Could you check a few things on this model? Use its own coordinates, in mm. Round coordinates to 2 decimals unless told otherwise and drop trailing zeros. Write each loop counter-clockwise with the first axis right and the second up, starting at its lowest first coordinate (ties: lowest second). Pieces come first, ordered by that corner, then holes. Notation, with made-up numbers: M 34,43 L 84,43 A8 cw 84,52 Z; hole C -29,-29.75 d5. An arc over 180 degrees is marked long. One line per item, written item: value. Start each with the question number.
(1) I want a section at B-B on y = 459. Please give me the cut outline in (x, z).
(2) I'm going to push flat-ended pins straight in: pin 1 Ø8 at (x, y) = (88.9, 12.7) entering from -Z; pin 2 Ø3 at (y, z) = (639, 2) entering from +X. Where does each tip first touch, or does it pass through?
(3) If I drill on L1, parallel to X at y = 1714.5, z = 3.5; L2, parallel to Y at x = 571.5, z = 5; L3, parallel to Y at x = 304.8, z = 4.25, over which ranges is the centre line in solid material (lowest first)?
(4) I want a section at A-A on z = 4.25. Count the separate pieces of the cut face and the enclosed holes in it, and give its area (3 significant figures).
```python
from build123d import *

# Parameters (mm, degrees)
SKETCH2_W                                       = 584.2
SKETCH2_H                                       = 1727.2
BOSS_EXTRUDE1_DEPTH                             = 6.35
CUT_EXTRUDE1_DEPTH                              = 1824.334802635
H_0_266_DIAMETER_HOLE1_D                        = 6.7564
FILLET1_R                                       = 6.35
SKETCH7_R                                       = 3.3782
CUT_EXTRUDE2_DEPTH                              = 12.7
CSK_FOR_10_FLAT_HEAD_MACHINE_SCREW1_D           = 5.6134
CSK_FOR_10_FLAT_HEAD_MACHINE_SCREW1_CSINK_D     = 9.779
CSK_FOR_10_FLAT_HEAD_MACHINE_SCREW1_CSINK_ANGLE = 82
SKETCH15_R                                      = 3.937
CUT_EXTRUDE3_DEPTH                              = 1824.334802635


with BuildPart() as part:
    # Sketch2 → Boss-Extrude1 (new body)
    with BuildSketch(Plane.XY):
        with Locations((292.1, 863.6)):
            Rectangle(SKETCH2_W, SKETCH2_H)
    extrude(amount=BOSS_EXTRUDE1_DEPTH)

    # Sketch3 → Cut-Extrude1 (cut, through all)
    with BuildSketch(Plane.XY.offset(6.35)):
        Polygon((584.2, 1098.55), (311.15, 1098.55), (311.15, 184.15), (431.8, 63.5), (431.8, 0), (584.2, 0), align=None)
    extrude(amount=-CUT_EXTRUDE1_DEPTH, mode=Mode.SUBTRACT)

    # H (0.266) Diameter Hole1 (through all)
    with Locations(Plane.XY.offset(6.35)):
        with Locations((12.7, 1714.5), (12.7, 1289.05), (12.7, 863.6), (12.7, 438.15), (12.7, 12.7), (571.5, 1111.25), (571.5, 1412.875), (571.5, 1714.5)):
            Hole(H_0_266_DIAMETER_HOLE1_D / 2)

    # Fillet1
    fillet1_edges = [part.edges().sort_by_distance(p)[0] for p in [
        (431.8, 0, 3.175),
        (431.8, 63.5, 3.175),
        (311.15, 184.15, 3.175),
        (311.15, 1098.55, 3.175),
        (0, 0, 3.175),
    ]]
    fillet(fillet1_edges, radius=FILLET1_R)

    # Sketch7 → Cut-Extrude2 (cut)
    with BuildSketch(Plane.XY.offset(6.35)):
        with Locations((88.9, 12.7)):
            Circle(SKETCH7_R)
        with Locations((342.9, 12.7)):
            Circle(SKETCH7_R)
    extrude(amount=-CUT_EXTRUDE2_DEPTH, mode=Mode.SUBTRACT)

    # CSK for #10 Flat Head Machine Screw1 (through all)
    with Locations(Plane(origin=(0, 0, 0), x_dir=(-1, 0, 0), z_dir=(0, 0, -1))):
        with Locations((-304.8, 342.9), (-304.8, 215.9), (-320.317182668, 166.002561211), (-410.119743879, 76.2)):
            CounterSinkHole(CSK_FOR_10_FLAT_HEAD_MACHINE_SCREW1_D / 2, CSK_FOR_10_FLAT_HEAD_MACHINE_SCREW1_CSINK_D / 2, counter_sink_angle=CSK_FOR_10_FLAT_HEAD_MACHINE_SCREW1_CSINK_ANGLE)

    # Sketch15 → Cut-Extrude3 (cut, through all)
    with BuildSketch(Plane.XY.offset(6.35)):
        with Locations((378.46762, 19.05)):
            Circle(SKETCH15_R)
        with Locations((378.46762, 76.2)):
            Circle(SKETCH15_R)
    extrude(amount=-CUT_EXTRUDE3_DEPTH, mode=Mode.SUBTRACT)


solid = part.part
```
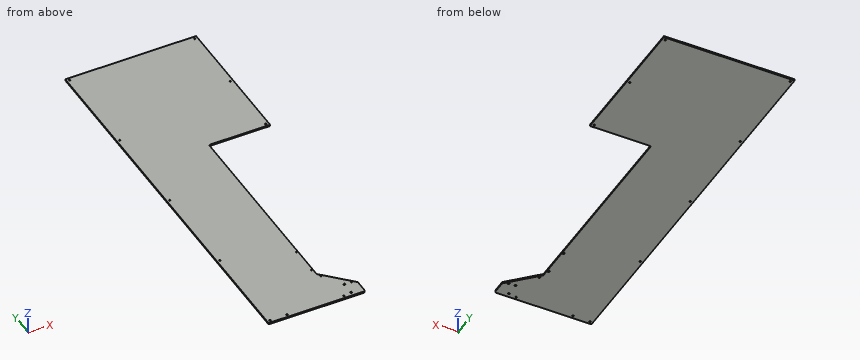
Found:
1. outline: M 0,0 L 311.15,0 L 311.15,6.35 L 0,6.35 Z
2. pin 1: stops at z = 0
2. pin 2: stops at x = 311.15
3. L1: x = 0 to 9.32, 16.08 to 568.12, 574.88 to 584.2
3. L2: y = 1098.55 to 1107.87, 1114.63 to 1409.5, 1416.25 to 1711.12, 1717.88 to 1727.2
3. L3: y = 0 to 213.09, 218.71 to 340.09, 345.71 to 1727.2
4. separate pieces: 1
4. enclosed holes: 16
4. area: 723,000 mm²
